```python
from build123d import *

# Parameters (mm, degrees)
SKETCH_R      = 7.5
EXTRUDE_DEPTH = 1


with BuildPart() as extrude_body:
    # Sketch → Extrude (new body)
    with BuildSketch(Plane.XY.offset(5)):
        Circle(SKETCH_R)
    extrude(amount=EXTRUDE_DEPTH)


with BuildPart() as fusion:
    # Sketch001 → Revolve (revolve)
    with BuildSketch(Plane.XZ):
        with BuildLine():
            Line((0, 0), (-10, 0))
            add(Edge.make_bspline(
                [(-9, 5), (-9.79, 3.99), (-10.13, 2.25), (-10, 0)],
                knots=[0, 0, 0, 0, 1, 1, 1, 1], degree=3))
            Line((-9, 5), (0, 5))
            Line((0, 5), (0, 0))
        make_face()
    revolve(axis=Axis((0, 0, 0), (0, 0, 1)))

    # Fusion: union Extrude body
    add(extrude_body.part)


solid = fusion.part
```
The listing builds one solid part. Answer for the finished solid, in the listing's coordinates (mm). A direction names the side the tool comes from. Give positions to 0.01 mm unless a question says otherwise; leave off trailing zeros. Loops run counter-clockwise (first coordinate to the right, second up) from the corner with the lowest first, then second, coordinate; pieces in that order, holes last. Notation, with made-up numbers: M 44.5,-21 L 70.5,-21 A16 cw 70.5,-12 Z; hole C -23.5,36 d6. An arc over 180 degrees is marked long. One line per item, written item: value.
1. Find the intervals of material crossed by probe 1 along Z at (x, y) = (7.25, -2.5); probe 2 along X at (y, z) = (-6.25, 5.5); probe 3 along Y at (x, z) = (1, 1.5), in increasing order.
Found:
probe 1: 0 to 5
probe 2: -4.15 to 4.15
probe 3: -9.96 to 9.96
2. Each of these flat-tipped pins is pushed along its axis until it touches: P1, Ø3, axis at y = 6.5, z = 5, coming from the -X side; P2, Ø1, axis at x = -2.5, z = 1, coming from the -Y side; P3, Ø2, axis at x = 2, z = 1.5, coming from the +Y side. Where does it stop, or does it pass through?
Found:
P1: x = -7.9
P2: y = -9.83
P3: y = 9.97
3. For faces 1 (the face through (-7.493, 0.33, 5.493)), 2 (the face through (0, 0, 0)), determine the directions among +Z, -Z, +X, -X, +Y, -Y from which every point of the face is accessible in a straight line to the end or side of a thin tool.
Found:
face 1: +Z
face 2: -Z, +X, -X, +Y, -Y
4. Section A-A on z = 5.25 is taken. Determine the outline of the cut face in (x, y).
Found:
outline: C 0,0 d15
